Verification items for the finished model (mm, model axes). A direction names the side the tool comes from. Coordinates: 2 decimals unless noted, no trailing zeros. Loops run counter-clockwise (first coordinate to the right, second up) from the corner with the lowest first, then second, coordinate; pieces in that order, holes last. Notation, with made-up numbers: (77.25, 48.5) -> (129.25, 48.5) arc R29 ccw to (129.25, 87.5) -> close; hole circle Ø9 at (76, 14). An arc over 180 degrees is marked (long way). Use CSV: the item, a comma, the result in double quotes. Start each with the question number.
```python
from build123d import *

# Parameters (mm, degrees)
SKETCH1_R           = 3.1
BOSS_EXTRUDE1_DEPTH = 15
SKETCH2_R           = 2.6
CUT_EXTRUDE2_DEPTH  = 32.912098558
CUT_EXTRUDE4_REACH  = 33.912
SKETCH3_W           = 7.5
SKETCH3_H           = 5
SKETCH4_W           = 7.5
SKETCH4_H           = 5.238037534
CUT_EXTRUDE5_DEPTH  = 5
FILLET1_R           = 1
FILLET2_R           = 3


with BuildPart() as part:
    # Sketch1 → Boss-Extrude1 (new body)
    with BuildSketch(Plane(origin=(0, 0, 0), x_dir=(0, 0, -1), z_dir=(1, 0, 0))):
        with BuildLine():
            Line((7.5, 2.5), (17.5, 2.5))
            Line((17.5, 2.5), (17.5, -2.5))
            Line((17.5, -2.5), (-17.5, -2.5))
            Line((-17.5, -2.5), (-17.5, 2.5))
            Line((-17.5, 2.5), (-7.5, 2.5))
            Line((-7.5, 2.5), (-7.5, 12.5))
            ThreePointArc((-7.5, 12.5), (-6.123724357, 16.830127019), (-2.5, 19.571067812))
            Line((-2.5, 19.571067812), (2.5, 19.571067812))
            ThreePointArc((2.5, 19.571067812), (6.123724357, 16.830127019), (7.5, 12.5))
            Line((7.5, 12.5), (7.5, 2.5))
        make_face()
        with Locations((0, 12.5)):
            Circle(SKETCH1_R, mode=Mode.SUBTRACT)
    extrude(amount=BOSS_EXTRUDE1_DEPTH)

    # Sketch2 → Cut-Extrude2 (cut, through all)
    with BuildSketch(Plane(origin=(0, 19.571067812, 0), x_dir=(1, 0, 0), z_dir=(0, 1, 0))):
        with Locations(Location((7.5, 12.5, 0), (0, 0, 270))):
            Circle(SKETCH2_R)
        with Locations(Location((7.5, -12.5, 0), (0, 0, 270))):
            Circle(SKETCH2_R)
    extrude(amount=-CUT_EXTRUDE2_DEPTH, mode=Mode.SUBTRACT)

    # Cut-Extrude4: up to this face of the body (flat: up to its plane)
    cut_extrude4_end = Plane(part.part.faces().sort_by_distance((7.5, 2.5, 17.319722436))[0])
    # Sketch3 → Cut-Extrude4 (cut, up to the picked face)
    with BuildSketch(Plane(origin=(0, 19.571067812, 0), x_dir=(1, 0, 0), z_dir=(0, 1, 0)), mode=Mode.PRIVATE) as cut_extrude4_sk1:
        with Locations((3.75, -5)):
            Rectangle(SKETCH3_W, SKETCH3_H)
    cut_extrude4_tool1 = split(extrude(cut_extrude4_sk1.sketch, amount=-CUT_EXTRUDE4_REACH, mode=Mode.PRIVATE), bisect_by=cut_extrude4_end, keep=Keep.BOTH, mode=Mode.PRIVATE)
    # Sketch3 → Cut-Extrude4 (cut, up to the picked face)
    with BuildSketch(Plane(origin=(0, 19.571067812, 0), x_dir=(1, 0, 0), z_dir=(0, 1, 0)), mode=Mode.PRIVATE) as cut_extrude4_sk2:
        with Locations((3.75, 5)):
            Rectangle(SKETCH3_W, SKETCH3_H)
    cut_extrude4_tool2 = split(extrude(cut_extrude4_sk2.sketch, amount=-CUT_EXTRUDE4_REACH, mode=Mode.PRIVATE), bisect_by=cut_extrude4_end, keep=Keep.BOTH, mode=Mode.PRIVATE)
    add(cut_extrude4_tool1.solids().sort_by(Axis((3.75, 19.571068, 5), (0, -1, 0)))[0], mode=Mode.SUBTRACT)
    add(cut_extrude4_tool2.solids().sort_by(Axis((3.75, 19.571068, -5), (0, -1, 0)))[0], mode=Mode.SUBTRACT)

    # Sketch4 → Cut-Extrude5 (cut)
    with BuildSketch(Plane.XY.offset(2.5)):
        Polygon((7.5, 8.666969722), (0, 2.5), (0, 10.666969722), (7.5, 10.666969722), align=None)
        with Locations((3.75, 16.952049045)):
            Rectangle(SKETCH4_W, SKETCH4_H)
    extrude(amount=-CUT_EXTRUDE5_DEPTH, mode=Mode.SUBTRACT)

    # Fillet1
    fillet1_edges = [part.edges().sort_by_distance(p)[0] for p in [
        (11.25, 2.5, 7.5),
        (11.25, 2.5, -7.5),
        (7.5, 2.5, -5),
        (3.75, 2.5, -2.5),
        (7.5, 2.5, 5),
        (3.75, 2.5, 2.5),
    ]]
    fillet(fillet1_edges, radius=FILLET1_R)

    # Fillet2
    fillet2_edges = [part.edges().sort_by_distance(p)[0] for p in [
        (0, 0, 17.5),
        (0, 0, -17.5),
        (15, 0, 17.5),
        (15, 0, -17.5),
    ]]
    fillet(fillet2_edges, radius=FILLET2_R)


solid = part.part
```
1. Cross-section at C-C, the plane z = -12.5. Record the boundary of the cut face in (x, y).
2. Depth check by flat-ended pin: pin 1 (4 mm diameter, centred on x = 6, y = 7, fed in from -Z); pin 2 (2.5 mm diameter, centred on x = 3, y = 5.5, fed in from +Z); pin 3 (2 mm diameter, centred on x = 12, y = 10, fed in from +Z). Enter the tip coordinate at first touch or a pass-through.
3. Release check for a two-part mould opening along Z. For faces 6 (the flat face through (6, 5, 2.5)), 7 (the cylindrical face through (6.5, 0, 14.9)), 8 (the cylindrical face through (6.5, 0, -10.1)), 9 (the flat face through (6, 2.5, -10)) record: released by +Z, released by -Z, zero draft, split by the parting line, or undercut.
4. Cross-section at A-A, the plane x = 8.5. Record the boundary of the cut face in (y, z), plus the area to 3 significant figures.
5. Cross-section at D-D, the plane y = 7.75. Record the boundary of the cut face in (x, z).
6. Cross-section at B-B, the plane z = 0. Record the boundary of the cut face in (x, y), plus the area to 3 significant figures.
7. Scan lines: line 1 (Z direction, x = 9.5, y = 12.5); line 2 (X direction, y = 0.9, z = -12.5); line 3 (Z direction, x = 5.75, y = -1.5). Record each from-to range of solid material in increasing order.
8. Set-up check for faces 1 (the flat face through (7.5, 11.6, 3.4)), 2 (the flat face through (6, 5, -2.5)), 3 (the flat face through (11, 8, 7.5)), 4 (the cylindrical face through (3.698, 2.785, 2.801)), 5 (the flat face through (11, 19.571, 0)): record each of +Z, -Z, +X, -X, +Y, -Y from which the full face is reachable in a straight line by a thin tool's end or side.
Solution:
1,outline,"(0, -2.5) -> (4.9, -2.5) -> (4.9, 2.5) -> (0, 2.5) -> close; (10.1, -2.5) -> (15, -2.5) -> (15, 2.5) -> (10.1, 2.5) -> close"
2,pin 1,"stops at z = -7.5"
2,pin 2,"stops at z = 2.5"
2,pin 3,"stops at z = 7.5"
3,face 6,"released by +Z"
3,face 7,"undercut"
3,face 8,"undercut"
3,face 9,"zero draft"
4,outline,"(-2.5, -17.5) -> (2.5, -17.5) -> (2.5, -14.9) -> (-2.5, -14.9) -> close; (-2.5, -10.1) -> (2.5, -10.1) -> (2.5, -8.5) arc R1 cw to (3.5, -7.5) -> (12.5, -7.5) arc R7.5 ccw to (19.57, -2.5) -> (19.57, 2.5) arc R7.5 ccw to (12.5, 7.5) -> (3.5, 7.5) arc R1 cw to (2.5, 8.5) -> (2.5, 10.1) -> (-2.5, 10.1) -> close; (-2.5, 14.9) -> (2.5, 14.9) -> (2.5, 17.5) -> (-2.5, 17.5) -> close; hole circle Ø6.2 at (12.5, 0)"
4,area,"334 mm2"
5,outline,"(6.38, -2.5) -> (7.5, -2.5) -> (7.5, -7.5) -> (15, -7.5) -> (15, 7.5) -> (7.5, 7.5) -> (7.5, 2.5) -> (6.38, 2.5) -> close"
6,outline,"(0, -2.5) -> (15, -2.5) -> (15, 9.4) -> (7.5, 9.4) -> (7.5, 8.67) -> (0, 2.5) -> close; (7.5, 15.6) -> (15, 15.6) -> (15, 19.57) -> (7.5, 19.57) -> close"
6,area,"180 mm2"
7,line 1,"z = -7.5 to -3.1, 3.1 to 7.5"
7,line 2,"x = 0 to 4.9, 10.1 to 15"
7,line 3,"z = -17.5 to -14.42, -10.58 to 10.58, 14.42 to 17.5"
8,face 1,"-X, +Y"
8,face 2,"-Z, -X, +Y"
8,face 3,"+Z, +X, -X, +Y"
8,face 4,"+Z, -X, +Y"
8,face 5,"+Z, -Z, +X, -X, +Y"
